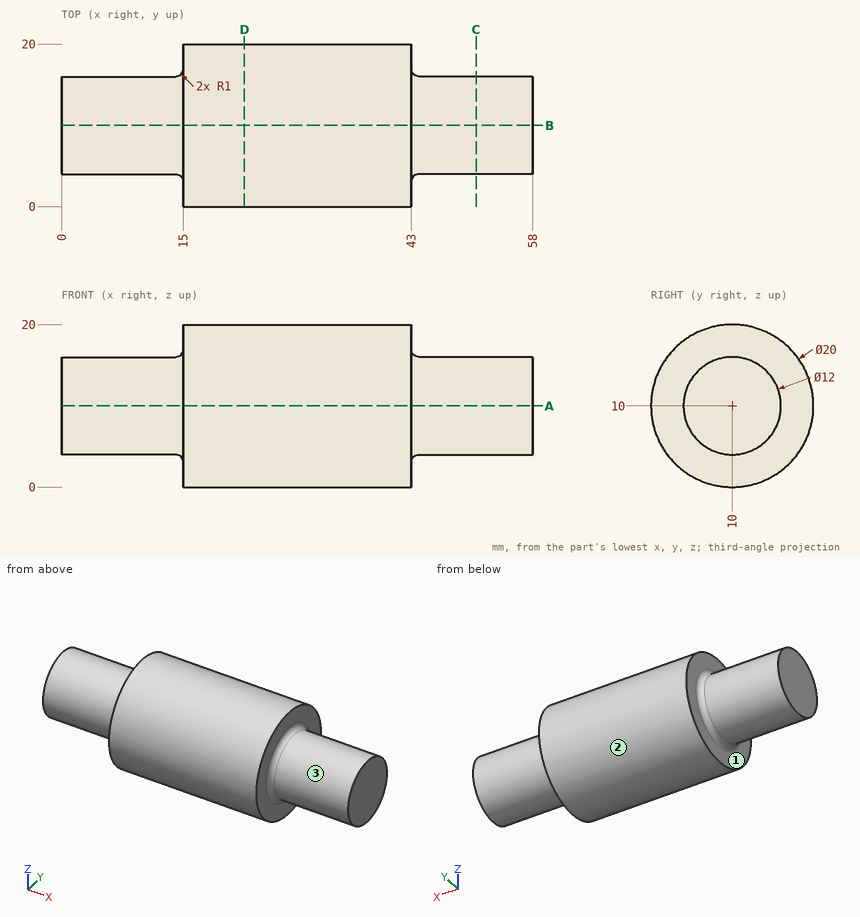
Can you work these out from the drawing? Everything is in mm from the part's minimum corner. A direction names the side the tool comes from. Give positions to 0.01 mm unless a question says otherwise; leave off trailing zeros. Loops run counter-clockwise (first coordinate to the right, second up) from the corner with the lowest first, then second, coordinate; pieces in that order, holes last. Notation, with made-up numbers: (83, 72) - (112, 72) arc R26 ccw to (112, 102) - close; hole circle Ø11 at (27.5, 17.5). An arc over 180 degrees is marked (long way). Answer as a JSON object with one key per item and string values.
Q1. If I drill on L1, parallel to Z at x = 38.5, y = 10.5; L2, parallel to X at y = 13.25, z = 1.5, over which ranges is the centre line in solid material (lowest first)?
Geometry says:
{"L1": "0.01 to 19.99", "L2": "15 to 43"}
Q2. Imagine slicing it at C-C on x = 51. Write out the boundary of the cut face in (y, z).
Geometry says:
{"outline": "circle Ø12 at (10, 10)"}
Q3. Which directions (+Z, -Z, +X, -X, +Y, -Y) give clear straight access to the entire face, cutting with the end or side of a thin tool? Please do the marked faces 1, 2 and 3.
Geometry says:
{"face 1": "-X", "face 2": "+X, -X", "face 3": "+X"}
Q4. Imagine slicing it at A-A on z = 10. Write out the boundary of the cut face in (x, y).
Geometry says:
{"outline": "(0, 4) - (14, 4) arc R1 cw to (15, 3) - (15, 0) - (43, 0) - (43, 3) arc R1 cw to (44, 4) - (58, 4) - (58, 16) - (44, 16) arc R1 cw to (43, 17) - (43, 20) - (15, 20) - (15, 17) arc R1 cw to (14, 16) - (0, 16) - close"}
Q5. Imagine slicing it at D-D on x = 22.5. Write out the boundary of the cut face in (y, z).
Geometry says:
{"outline": "circle Ø20 at (10, 10)"}
Q6. Will these pins go through, and if not, where does the flat tip stop? P1, Ø5, axis at x = 27.5, y = 2.5, coming from the +Z side; P2, Ø6, axis at x = 48.5, z = 14.5, coming from the -Y side.
Geometry says:
{"P1": "z = 18.66", "P2": "y = 4.19"}
